The model under review builds one solid part; all positions refer to its coordinate system, in mm. A direction names the side the tool comes from. Round coordinates to 2 decimals unless told otherwise and drop trailing zeros. Write each loop counter-clockwise with the first axis right and the second up, starting at its lowest first coordinate (ties: lowest second). Pieces come first, ordered by that corner, then holes. Notation, with made-up numbers: M 89,-26.5 L 134,-26.5 A23 ccw 134,3.5 Z; hole C 82,-17 d2. An arc over 180 degrees is marked long. One line per item, written item: value. Start each with the question number.
1) Tool access review of faces 5 (the face through (15, 6.2, 3)), 6 (the face through (29.5, 3, 3)), 7 (the face through (15, 0.2, 3)), 8 (the face through (1, 3, 3)): name each direction out of +Z, -Z, +X, -X, +Y, -Y from which nothing blocks a thin tool from reaching the whole face with its end or side.
2) Wall thickness on probe 1 along Y at (x, z) = (3.7, 0.4); probe 2 along Y at (x, z) = (26.5, 0.9); probe 3 along Z at (x, y) = (4.5, 17): over which ranges is each line inside the solid? List them lowest first.
3) Take a section at B-B, the plane y = 9.8. Write out the cut boundary in (x, z), and give its area (3 significant figures).
4) Take a section at A-A, the plane x = 26.5. Write out the cut boundary in (y, z), and give its area (3 significant figures).
5) For P1, Ø1.5, axis at y = 3.5, z = 2.5, coming from the +X side; P2, Ø2.5, axis at x = 10.5, z = 3.5, coming from the +Y side; P3, Ø2.5, axis at y = 2.5, z = 3.5, coming from the -X side, all flat-tipped, find the tip position at first contact; note any pin that passes through.
6) Take a section at D-D, the plane x = 12. Write out the cut boundary in (y, z), and give its area (3 significant figures).
7) Mouldability with a two-part tool opening along Y and no side actions: class faces 1 (the face through (15, 0, 1)), 2 (the face through (3.895, 26.987, 0.789)), 3 (the face through (15, 30.5, 1)), 4 (the face through (30.5, 15, 1)) as +Y half, -Y half, draft (parallel to the pull), parting line (faces both ways), or undercut.
8) Take a section at C-C, the plane z = 0.95. Write out the cut boundary in (x, y).
from build123d import *

# Parameters (mm, degrees)
SKETCH1_W             = 30.5
SKETCH1_H             = 30.5
BOSS_EXTRUDE1_DEPTH   = 1.6
F_3_0MM_DOWEL_HOLE1_D = 3
SKETCH4_W             = 28.5
SKETCH4_H             = 6
BOSS_EXTRUDE2_DEPTH   = 3


with BuildPart() as part:
    # Sketch1 → Boss-Extrude1 (new body)
    with BuildSketch(Plane.XY):
        with Locations((15.25, 15.25)):
            Rectangle(SKETCH1_W, SKETCH1_H)
    extrude(amount=BOSS_EXTRUDE1_DEPTH)

    # Ø3.0mm Dowel Hole1 (through all)
    with Locations(Plane.XY.offset(1.6)):
        with Locations((3.7, 25.5), (26.5, 9.8)):
            Hole(F_3_0MM_DOWEL_HOLE1_D / 2)

    # Sketch4 → Boss-Extrude2 (add)
    with BuildSketch(Plane.XY.offset(1.6)):
        with Locations((15.25, 3.2)):
            Rectangle(SKETCH4_W, SKETCH4_H)
    extrude(amount=BOSS_EXTRUDE2_DEPTH)


solid = part.part
Checked values:
1. face 5: +Z, +X, -X, +Y
1. face 6: +Z, +X, +Y, -Y
1. face 7: +Z, +X, -X, -Y
1. face 8: +Z, -X, +Y, -Y
2. probe 1: y = 0 to 24, 27 to 30.5
2. probe 2: y = 0 to 8.3, 11.3 to 30.5
2. probe 3: z = 0 to 1.6
3. outline: M 0,0 L 25,0 L 25,1.6 L 0,1.6 Z; M 28,0 L 30.5,0 L 30.5,1.6 L 28,1.6 Z
3. area: 44.0 mm2
4. outline: M 0,0 L 8.3,0 L 8.3,1.6 L 6.2,1.6 L 6.2,4.6 L 0.2,4.6 L 0.2,1.6 L 0,1.6 Z; M 11.3,0 L 30.5,0 L 30.5,1.6 L 11.3,1.6 Z
4. area: 62.0 mm2
5. P1: stops at x = 29.5
5. P2: stops at y = 6.2
5. P3: stops at x = 1
6. outline: M 0,0 L 30.5,0 L 30.5,1.6 L 6.2,1.6 L 6.2,4.6 L 0.2,4.6 L 0.2,1.6 L 0,1.6 Z
6. area: 66.8 mm2
7. face 1: -Y half
7. face 2: undercut
7. face 3: +Y half
7. face 4: draft
8. outline: M 0,0 L 30.5,0 L 30.5,30.5 L 0,30.5 Z; hole C 3.7,25.5 d3; hole C 26.5,9.8 d3
